```python
from build123d import *

# Parameters (mm, degrees)
SKETCH_2_R      = 6
EXTRUDE_1_DEPTH = 6
EXTRUDE_2_DEPTH = 11


with BuildPart() as part:
    # 草图1 → 旋转1 (revolve)
    with BuildSketch(Plane(origin=(0, 0, 0), x_dir=(1, 0, 0), z_dir=(0, 1, 0)), mode=Mode.PRIVATE) as revolve_1_sk:
        Polygon((0, 18.5), (0, 0), (53, 0), (53, 7), (49, 7), (49, 3), (46, 3), (46, 16.4), (22, 16.4), (22, 18.5), align=None)
    revolve(revolve_1_sk.sketch.rotate(Axis((0, 0, 0), (1, 0, 0)), 180), axis=Axis((0, 0, 0), (1, 0, 0)))

    # 草图2 → 凸台-拉伸1 (add)
    with BuildSketch(Plane.ZY):
        with Locations((0, 7)):
            Circle(SKETCH_2_R)
    extrude(amount=EXTRUDE_1_DEPTH)

    # 草图3 → 凸台-拉伸2 (add)
    with BuildSketch(Plane.ZY.offset(6)):
        with BuildLine():
            Line((-1.8, 9.4), (1.8, 9.4))
            ThreePointArc((1.8, 9.4), (0, 4), (-1.8, 9.4))
        make_face()
    extrude(amount=EXTRUDE_2_DEPTH)


solid = part.part
```
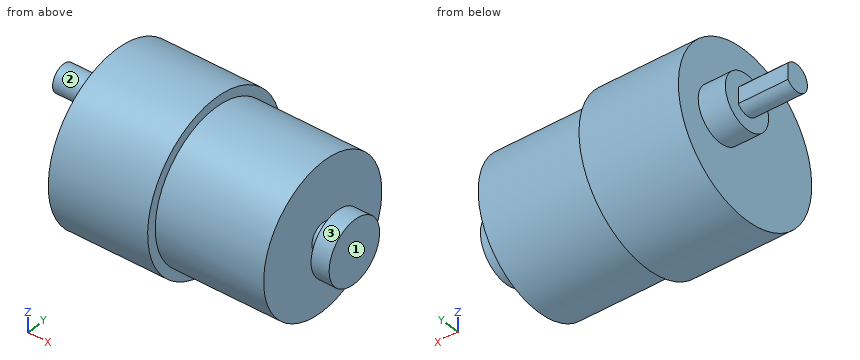
For this review, take the finished solid that the model builds, in its own axes (mm). Face numbers are marked on the shaded views. A direction names the side the tool comes from. Give positions to 0.01 mm unless a question says otherwise; leave off trailing zeros. Write each loop counter-clockwise with the first axis right and the second up, starting at its lowest first coordinate (ties: lowest second). Pieces come first, ordered by that corner, then holes. Notation, with made-up numbers: M 64,88.25 L 79,88.25 A25 cw 79,100.25 Z; hole C -37,-10 d8. An arc over 180 degrees is marked long. Answer as a JSON object with one key per item and string values. Group by question number.
Item 1: Consider section D-D on z = 11.5. Write out the cut boundary in (x, y), plus the area to 3 significant figures.
Item 2: Consider section C-C on x = 24.5. Write out the cut boundary in (y, z).
Item 3: For probe 1 along X at (y, z) = (-6, -3); probe 2 along X at (y, z) = (16, 4); probe 3 along Y at (x, z) = (16.5, 0), list the stretches that pass through material, from the lowest coordinate up. Write a range as [from, to].
Item 4: Tool access review of the marked faces 1, 2 and 3: name each direction out of +Z, -Z, +X, -X, +Y, -Y from which nothing blocks a thin tool from reaching the whole face with its end or side.
Item 5: Consider section A-A on z = 0. Write out the cut boundary in (x, y).
Item 6: For pin 1 Ø10 at (y, z) = (0.5, -7.5) entering from -X; pin 2 Ø1.8 at (x, z) = (-11.5, 0.5) entering from +Y; pin 3 Ø6 at (x, z) = (6.5, 14.5) entering from -Y, all flat-tipped, find the tip position at first contact; note any pin that passes through.
Item 7: Consider section B-B on y = 0. Write out the cut boundary in (x, z), plus the area to 3 significant figures.
Check result:
{
 "1": {"outline": "M 0,-14.49 L 22,-14.49 L 22,-11.69 L 46,-11.69 L 46,11.69 L 22,11.69 L 22,14.49 L 0,14.49 Z", "area": "1,200 mm^2"},
 "2": {"outline": "C 0,0 d32.8"},
 "3": {"probe 1": "x = [0, 46], [49, 53]", "probe 2": "x = [0, 22]", "probe 3": "y = [-18.5, 18.5]"},
 "4": {"face 1": "+Z, -Z, +X, +Y, -Y", "face 2": "-X", "face 3": "+X"},
 "5": {"outline": "M -17,4 L -6,4 L -6,1 L 0,1 L 0,-18.5 L 22,-18.5 L 22,-16.4 L 46,-16.4 L 46,-3 L 49,-3 L 49,-7 L 53,-7 L 53,7 L 49,7 L 49,3 L 46,3 L 46,16.4 L 22,16.4 L 22,18.5 L 0,18.5 L 0,13 L -6,13 L -6,9.4 L -17,9.4 Z"},
 "6": {"pin 1": "stops at x = -6", "pin 2": "stops at y = 9.4", "pin 3": "stops at y = -14.49"},
 "7": {"outline": "M 0,-18.5 L 22,-18.5 L 22,-16.4 L 46,-16.4 L 46,-3 L 49,-3 L 49,-7 L 53,-7 L 53,7 L 49,7 L 49,3 L 46,3 L 46,16.4 L 22,16.4 L 22,18.5 L 0,18.5 Z", "area": "1,680 mm^2"}
}
